```python
from build123d import *

# Parameters (mm, degrees)
SKETCH1_R           = 2.1463
BOSS_EXTRUDE1_DEPTH = 2.3622
SKETCH2_R           = 1.5875
CUT_EXTRUDE1_DEPTH  = 10
SKETCH4_R           = 6
SKETCH4_R_2         = 5.999999938
CUT_EXTRUDE3_DEPTH  = 10
SKETCH6_R           = 1
CUT_EXTRUDE4_DEPTH  = 10
CIRPATTERN2_COUNT   = 3
SKETCH7_R           = 1.14935
CUT_EXTRUDE5_DEPTH  = 2.54
CIRPATTERN3_COUNT   = 3
SKETCH8_W           = 13.106463283
SKETCH8_H           = 11.477303128
CUT_EXTRUDE6_DEPTH  = 2.54


with BuildPart() as part:
    # Sketch1 → Boss-Extrude1 (new body)
    with BuildSketch(Plane(origin=(0, 0, 0), x_dir=(1, 0, 0), z_dir=(0, 1, 0))):
        with BuildLine():
            Line((-30, 44.45), (-30, 70.045984896))
            ThreePointArc((-30, 70.045984896), (-65.991135768, 38.1), (-75.661602353, -9.042230334))
            Line((-75.661602353, -9.042230334), (-53.494829198, 3.755762114))
            Line((-53.494829198, 3.755762114), (-23.494829198, -48.205762114))
            Line((-23.494829198, -48.205762114), (-45.661602353, -61.003754561))
            ThreePointArc((-45.661602353, -61.003754561), (0, -76.2), (45.661602353, -61.003754561))
            Line((45.661602353, -61.003754561), (23.494829198, -48.205762114))
            Line((23.494829198, -48.205762114), (53.494829198, 3.755762114))
            Line((53.494829198, 3.755762114), (75.661602353, -9.042230334))
            ThreePointArc((75.661602353, -9.042230334), (65.991135768, 38.1), (30, 70.045984896))
            Line((30, 70.045984896), (30, 44.45))
            Line((30, 44.45), (-30, 44.45))
        make_face()
        with Locations(Location((-41.747414599, 24.102881057, 0), (0, 0, 270))):
            Circle(SKETCH1_R, mode=Mode.SUBTRACT)
        with Locations(Location((41.747414599, 24.102881057, 0), (0, 0, 270))):
            Circle(SKETCH1_R, mode=Mode.SUBTRACT)
        with Locations(Location((0, -53.205762114, 0), (0, 0, 90))):
            Circle(SKETCH1_R, mode=Mode.SUBTRACT)
    extrude(amount=BOSS_EXTRUDE1_DEPTH)

    # Sketch2 → Cut-Extrude1 (cut)
    with BuildSketch(Plane(origin=(0, 2.3622, 0), x_dir=(1, 0, 0), z_dir=(0, 1, 0))):
        with Locations(Location((18.25625, -68.58, 0), (0, 0, 270))):
            Circle(SKETCH2_R)
        with Locations(Location((-18.25625, -68.58, 0), (0, 0, 270))):
            Circle(SKETCH2_R)
    cut_extrude1 = extrude(amount=-CUT_EXTRUDE1_DEPTH, mode=Mode.SUBTRACT)

    # Sketch4 → Cut-Extrude3 (cut)
    with BuildSketch(Plane(origin=(0, 2.3622, 0), x_dir=(1, 0, 0), z_dir=(0, 1, 0))):
        with Locations(Location((0, -41.205762114, 0), (0, 0, 270))):
            Circle(SKETCH4_R)
        with Locations(Location((-31.095337868, 17.952901689, 0), (0, 0, 270))):
            Circle(SKETCH4_R_2)
    extrude(amount=-CUT_EXTRUDE3_DEPTH, mode=Mode.SUBTRACT)

    # Sketch6 → Cut-Extrude4 (cut)
    with BuildSketch(Plane.XZ):
        with Locations(Location((0, 0, 0), (0, 0, 270))):
            Circle(SKETCH6_R)
    extrude(amount=-CUT_EXTRUDE4_DEPTH, mode=Mode.SUBTRACT)

    # CirPattern2: Cut-Extrude1 ×3 about axis
    cirpattern2_axis = Axis((0, 0, 0), (0, 1, 0))
    for i in range(1, CIRPATTERN2_COUNT):
        add(cut_extrude1.rotate(cirpattern2_axis, i * 360 / CIRPATTERN2_COUNT), mode=Mode.SUBTRACT)

    # Sketch7 → Cut-Extrude5 (cut)
    with BuildSketch(Plane.XZ):
        with Locations(Location((8.73125, -31.75, 0), (0, 0, 270))):
            Circle(SKETCH7_R)
        with Locations(Location((-8.73125, -31.75, 0), (0, 0, 270))):
            Circle(SKETCH7_R)
    cut_extrude5 = extrude(amount=-CUT_EXTRUDE5_DEPTH, mode=Mode.SUBTRACT)

    # CirPattern3: Cut-Extrude5 ×3 about axis
    cirpattern3_axis = Axis((0, 0, 0), (0, 1, 0))
    for i in range(1, CIRPATTERN3_COUNT):
        add(cut_extrude5.rotate(cirpattern3_axis, i * 360 / CIRPATTERN3_COUNT), mode=Mode.SUBTRACT)

    # Sketch8 → Cut-Extrude6 (cut)
    with BuildSketch(Plane(origin=(0, 2.3622, 0), x_dir=(1, 0, 0), z_dir=(0, 1, 0))):
        with Locations((23.446768359, 38.711348436)):
            Rectangle(SKETCH8_W, SKETCH8_H)
    extrude(amount=-CUT_EXTRUDE6_DEPTH, mode=Mode.SUBTRACT)


solid = part.part
```
Work out the finished part from the listing and answer in its coordinate system (mm). A direction names the side the tool comes from. Coordinates: 2 decimals unless noted, no trailing zeros. Loops run counter-clockwise (first coordinate to the right, second up) from the corner with the lowest first, then second, coordinate; pieces in that order, holes last. Notation, with made-up numbers: (-1, 7.5) - (55, 7.5) arc R12 ccw to (55, 23.5) - close; hole circle Ø8 at (18.5, 60). An arc over 180 degrees is marked (long way). Use a Markdown table: item, result.
Item 1: Find section D-D, the plane z = 37. Determine the outline of the cut face in (x, y).
Evaluation:
| item | result |
|---|---|
| outline | (-29.96, 0) - (-4.28, 0) - (-4.28, 2.36) - (-29.96, 2.36) - close; (4.28, 0) - (29.96, 0) - (29.96, 2.36) - (4.28, 2.36) - close |
Item 2: Consider probe 1 along X at (y, z) = (1.8, 68.58); probe 2 along X at (y, z) = (1.6, 7); probe 3 along Z at (x, y) = (-36.5, 2.2). Determine where each line is inside the solid, lowest interval first. Write a range as from..to.
Evaluation:
| item | result |
|---|---|
| probe 1 | x = -33.21..-19.84, -16.67..16.67, 19.84..33.21 |
| probe 2 | x = -75.88..-72.12, -47.28..47.28, 72.12..75.88 |
| probe 3 | z = -66.89..-20.56, -15.35..25.68, 55.71..66.89 |
Item 3: For faces 4 (the flat face through (-34.4, 1.2, 54.5)), 5 (the flat face through (-38.705, 1.165, 21.861)), 6 (the flat face through (64.42, 1.16, 2.55)), 7 (the flat face through (34.733, 1.165, 54.694)), determine the directions among +Z, -Z, +X, -X, +Y, -Y from which every point of the face is accessible in a straight line to the end or side of a thin tool.
Evaluation:
| item | result |
|---|---|
| face 4 | -X, +Y, -Y |
| face 5 | +Y, -Y |
| face 6 | +Z, +Y, -Y |
| face 7 | +X, +Y, -Y |
Item 4: Find section A-A, the plane x = -28. Determine the outline of the cut face in (y, z).
Evaluation:
| item | result |
|---|---|
| outline | (0, -44.45) - (2.36, -44.45) - (2.36, -23.09) - (0, -23.09) - close; (0, -12.81) - (2.36, -12.81) - (2.36, 40.4) - (0, 40.4) - close; (0, 50.81) - (2.36, 50.81) - (2.36, 70.87) - (0, 70.87) - close |
Item 5: Find section C-C, the plane y = 1. State how many separate pieces and enclosed holes the cut face has, and give its area (3 significant figures).
Evaluation:
| item | result |
|---|---|
| separate pieces | 1 |
| enclosed holes | 18 |
| area | 12,400 mm2 |
Item 6: Find section B-B, the plane z = -57. Determine the outline of the cut face in (x, y), and give its area (3 significant figures).
Evaluation:
| item | result |
|---|---|
| outline | (-50.57, 0) - (-30, 0) - (-30, 2.36) - (-50.57, 2.36) - close; (30, 0) - (50.57, 0) - (50.57, 2.36) - (30, 2.36) - close |
| area | 97.2 mm2 |
Item 7: Given pin 1 Ø3 at (x, z) = (50.26, -50.1) entering from +Y; pin 2 Ø1.2 at (x, y) = (21, 1.5) entering from -Z, each flat-ended and moving along its own axis, determine where each tip first touches the part or whether it passes through.
Evaluation:
| item | result |
|---|---|
| pin 1 | passes through |
| pin 2 | stops at z = -32.97 |
Item 8: The mould has two halves that part along Z. Classify faces 1 (the flat face through (-1, 0, 2)), 2 (the cylindrical face through (-49.19, 1.2, -51.27)), 3 (the flat face through (-64.73, 1.16, 2.73)): +Z half, -Z half, draft (parallel to the pull), parting line (faces both ways), or undercut.
Evaluation:
| item | result |
|---|---|
| face 1 | draft |
| face 2 | undercut |
| face 3 | +Z half |
